from build123d import *

# Parameters (mm, degrees)
SKETCH_1_W          = 60
SKETCH_1_H          = 20
SKETCH_1_W_2        = 30
SKETCH_1_H_2        = 35
EXTRUDE_1_DEPTH     = 30
SKETCH_2_R          = 5
CUT_EXTRUDE_1_DEPTH = 87.746757864
SKETCH_3_W          = 5
SKETCH_3_H          = 35
CUT_EXTRUDE_2_DEPTH = 87.746757864
FILLET_1_R          = 2


with BuildPart() as part:
    # 草图1 → 凸台-拉伸1 (new body)
    with BuildSketch(Plane.XY):
        with Locations((30, 10)):
            Rectangle(SKETCH_1_W, SKETCH_1_H)
        with Locations((45, 37.5)):
            Rectangle(SKETCH_1_W_2, SKETCH_1_H_2)
    extrude(amount=EXTRUDE_1_DEPTH)

    # 草图2 → 切除-拉伸1 (cut, through all)
    with BuildSketch(Plane.XY.offset(30)):
        with Locations((15, 10)):
            Circle(SKETCH_2_R)
        with Locations((45, 10)):
            Circle(SKETCH_2_R)
        with Locations((45, 40)):
            Circle(SKETCH_2_R)
    extrude(amount=-CUT_EXTRUDE_1_DEPTH, mode=Mode.SUBTRACT)

    # 草图3 → 切除-拉伸2 (cut, through all)
    with BuildSketch(Plane.XY.offset(30)):
        with Locations((32.5, 37.5)):
            Rectangle(SKETCH_3_W, SKETCH_3_H)
        Polygon((60, 20), (60, 55), (55, 55), (55, 20), (55, 0), (60, 0), align=None)
    extrude(amount=-CUT_EXTRUDE_2_DEPTH, mode=Mode.SUBTRACT)

    # 圆角1
    fillet_1_edges = [part.edges().sort_by_distance(p)[0] for p in [
        (27.5, 0, 0),
        (0, 0, 15),
        (0, 20, 15),
        (17.5, 20, 30),
        (0, 10, 30),
        (45, 55, 0),
        (45, 55, 30),
        (55, 27.5, 0),
        (55, 0, 15),
        (55, 55, 15),
        (55, 27.5, 30),
        (27.5, 0, 30),
        (35, 37.5, 0),
        (35, 55, 15),
        (35, 20, 15),
        (35, 37.5, 30),
        (0, 10, 0),
        (17.5, 20, 0),
    ]]
    fillet(fillet_1_edges, radius=FILLET_1_R)


solid = part.part
CAD build for the part. Positions are in the model's coordinates, mm. A direction names the side the tool comes from. Round coordinates to 2 decimals unless told otherwise and drop trailing zeros. Order: outer loops, then holes, each group sorted by start corner. A loop starts at its lowest first (then second) coordinate and runs counter-clockwise, first axis right, second up. Notation, with made-up numbers: M 63.5,19.5 L 73.5,19.5 A13 ccw 73.5,23.5 Z; hole C 78,-2.75 d3. An arc over 180 degrees is marked long. Use one line per item in the form item = value.
Q1. Which spindle directions (+Z, -Z, +X, -X, +Y, -Y) get a long thin tool onto all of the face, cutting with end or side? Do faces 5 (the cylindrical face through (35.57, 37.72, 0.6)), 6 (the cylindrical face through (45.11, 54.4, 29.43)), 7 (the cylindrical face through (35.6, 37.72, 29.43)). Say none if no direction does.
Recorded:
face_5 = -Z, -X, +Y
face_6 = +Z, +X, -X, +Y
face_7 = +Z, -X, +Y
Q2. Saw through at D-D on x = 15. Give the cut face in (y, z), then the cut area to 3 significant figures.
Recorded:
outline = M 0,2 A2 ccw 2,0 L 5,0 L 5,30 L 2,30 A2 ccw 0,28 Z; M 15,0 L 18,0 A2 ccw 20,2 L 20,28 A2 ccw 18,30 L 15,30 Z
area = 297 mm^2
Q3. Saw through at A-A on y = 40. Give the cut face in (x, z).
Recorded:
outline = M 35,2 A2 ccw 37,0 L 40,0 L 40,30 L 37,30 A2 ccw 35,28 Z; M 50,0 L 53,0 A2 ccw 55,2 L 55,28 A2 ccw 53,30 L 50,30 Z
Q4. Flat gauge pins, fed straight in: P1, Ø3, axis at y = 37, z = 17, coming from the -X side; P2, Ø6, axis at x = 45, y = 10, coming from the +Z side; P3, Ø6, axis at x = 19.5, z = 17.5, coming from the +Y side; P4, Ø11.5, axis at x = 15, y = 10, coming from the -Z side. Where does each tip first touch, or does it go through?
Recorded:
P1 = 35
P2 = through
P3 = 20
P4 = 0
Q5. Saw through at B-B on x = 45. Give the cut face in (y, z).
Recorded:
outline = M 0,2 A2 ccw 2,0 L 5,0 L 5,30 L 2,30 A2 ccw 0,28 Z; M 15,0 L 35,0 L 35,30 L 15,30 Z; M 45,0 L 53,0 A2 ccw 55,2 L 55,28 A2 ccw 53,30 L 45,30 Z
Q6. Probe L1, parallel to Y at x = 45, z = 17.25; L2, parallel to Y at x = 41.5, z = 8; L3, parallel to Y at x = 15, z = 13. List the from-to ranges inside material, lowest first.
Recorded:
L1 = 0 to 5, 15 to 35, 45 to 55
L2 = 0 to 6.43, 13.57 to 36.43, 43.57 to 55
L3 = 0 to 5, 15 to 20
Q7. Saw through at C-C on y = 6. Give the cut face in (x, z), then the cut area to 3 significant figures.
Recorded:
outline = M 0,2 A2 ccw 2,0 L 12,0 L 12,30 L 2,30 A2 ccw 0,28 Z; M 18,0 L 42,0 L 42,30 L 18,30 Z; M 48,0 L 53,0 A2 ccw 55,2 L 55,28 A2 ccw 53,30 L 48,30 Z
area = 1,290 mm^2
Q8. Two-plate mould, pull along X, no slides. Class faces 1 (the cylindrical face through (19.77, 11.5, 15.21)), 2 (the cylindrical face through (27.86, 0.6, 0.57)), 3 (the cylindrical face through (0.57, 10.11, 0.6)), 4 (the cylindrical face through (54.4, 54.43, 14.82)): +X half, -X half, draft (parallel to the pull), parting line (faces both ways), or undercut.
Recorded:
face_1 = undercut
face_2 = draft
face_3 = -X half
face_4 = +X half
